Source: CAD feature listing. Evaluate the final solid. Frame: model axes, mm. A direction names the side the tool comes from. Round coordinates to 2 decimals unless told otherwise and drop trailing zeros. Write each loop counter-clockwise with the first axis right and the second up, starting at its lowest first coordinate (ties: lowest second). Pieces come first, ordered by that corner, then holes.
Autodesk Inventor part; units mm, degrees
ref_plane "YZ Plane" through (0, 0, 0) normal (1, 0, 0) x (0, 1, 0)
ref_plane "XZ Plane" through (0, 0, 0) normal (0, 1, 0) x (-1, 0, 0)
ref_plane "XY Plane" through (0, 0, 0) normal (0, 0, 1) x (1, 0, 0)
sketch "Sketch1" plane through (0, 0, 0) normal (0, 1, 0) x (-1, 0, 0)
  point P0 (0, 0)
sketch "Sketch2" plane through (0, 0, 0) normal (0, 1, 0) x (-1, 0, 0)
  circle A0 centre (0, 0) radius 5
  circle A1 centre (0, 0) radius 7
  line L0 (-0.0083, 4) -> (-10.0083, 4)
  line L1 (-10.0083, 4) -> (-10.0083, -4)
  line L2 (-10.0083, -4) -> (-0.0083, -4)
  line L3 (-0.0083, -4) -> (-0.0083, 4)
  point P0 (-3, -4)
  point P1 (-5.7446, -4)
  point P2 (-5.7446, 4)
  point P3 (-3, 4)
  dimension "d0" = 10
  dimension "d1" = 14
  dimension "d2" = 10
  dimension "d3" = 8
  dimension "d4" = 3
extrude "Extrusion1" add sketch "Sketch2" along normal blind 30 contours A0 L0 A1 L2 picked at (-4.4748, -4.4019)
sketch "Sketch3" plane through (0, 0, 0) normal (0, -1, 0) x (1, 0, 0)
  circle A0 centre (0, 0) radius 15
  dimension "d7" = 30
extrude "Extrusion2" add sketch "Sketch3" along normal blind 3
properties part number "fsrBase"
Q1. Set-up query: faces 1 (the face through (4, 15, 4)), 2 (the face through (-5, 30, 2)), 3 (the face through (-7, 15, 0)). Return all of +Z, -Z, +X, -X, +Y, -Y with unobstructed straight access to the full face (end or side cutting, diameter ignored); none if empty.
Q2. Line query: line 1 (Z direction, x = 0, y = 17); line 2 (X direction, y = 9.25, z = 0); line 3 (Y direction, x = 9.5, z = 7.5). Output: solid intervals per line, ascending.
Q3. Section query D-D, the plane z = -5.5. Output: boundary loops of the cut face in (x, y), and give its area (3 significant figures).
Q4. Mould query, pull axis Z, two halves, no side actions, for faces 4 (the face through (0, -3, 0)), 5 (the face through (-14.985, -1.479, -0.66)), 6 (the face through (-5, 15, 0)), 7 (the face through (4, 15, -4)). Classes: pulls with the +Z half, pulls with the -Z half, needs draft (parallel to the pull), parting line crosses it, or undercut.
Q5. Section query B-B, the plane z = 0. Output: boundary loops of the cut face in (x, y), and give its area (3 significant figures).
Q6. Section query C-C, the plane y = 7. Output: boundary loops of the cut face in (x, z), and give its area (3 significant figures).
Q7. Section query A-A, the plane x = 0. Output: boundary loops of the cut face in (y, z).
Q8. Pin query (flat end, axial travel): P1, Ø1, axis at x = -4.5, y = 2.5, coming from the -Z side; P2, Ø2, axis at x = 4.5, y = 16.5, coming from the +Z side; P3, Ø10, axis at x = 7.5, y = 10.5, coming from the -Z side. Return the tip coordinate at first contact, or that it passes through.
Filled in:
1. face 1: +X, +Y
1. face 2: +Z, -Z, +X, -X, +Y
1. face 3: +Y
2. line 1: z = -7 to -5, 5 to 7
2. line 2: x = -7 to -5
2. line 3: y = -3 to 0
3. outline: (-13.96, -3) - (13.96, -3) - (13.96, 0) - (4.33, 0) - (4.33, 30) - (-4.33, 30) - (-4.33, 0) - (-13.96, 0) - close
3. area: 344 mm2
4. face 4: needs draft
4. face 5: parting line crosses it
4. face 6: undercut
4. face 7: undercut
5. outline: (-15, -3) - (15, -3) - (15, 0) - (-5, 0) - (-5, 30) - (-7, 30) - (-7, 0) - (-15, 0) - close
5. area: 150 mm2
6. outline: (3, -4) arc R5 cw (long way) to (3, 4) - (5.74, 4) arc R7 ccw (long way) to (5.74, -4) - close
6. area: 57.8 mm2
7. outline: (-3, -15) - (0, -15) - (0, -7) - (30, -7) - (30, -5) - (0, -5) - (0, 5) - (30, 5) - (30, 7) - (0, 7) - (0, 15) - (-3, 15) - close
8. P1: stops at z = -5.74
8. P2: stops at z = 6.06
8. P3: stops at z = -6.54
